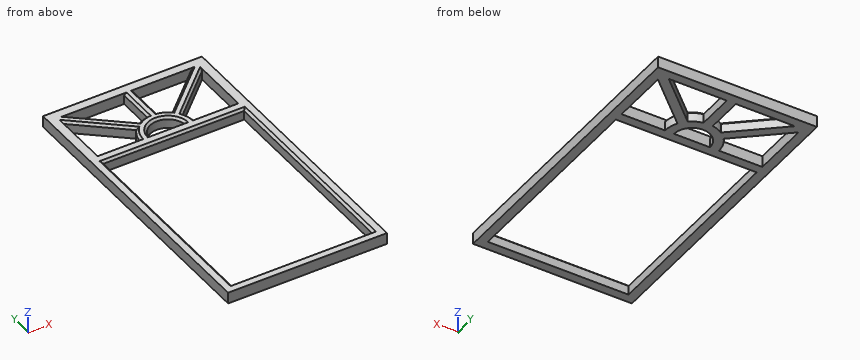
from build123d import *

# Parameters (mm, degrees)
F0_W     = 700
F0_H     = 1300
F0_W_2   = 620
F0_H_2   = 900
F1_DEPTH = 50
F2_SIZE  = 10


# Not quite as in the source:
# - a feature names something its author has since deleted; it is built from what else it names


with BuildPart() as f1:
    # F0 (on Top) → F1 (new body)
    with BuildSketch(Plane.XY):
        with Locations((-12.4809433535, 115.0203361814)):
            Rectangle(F0_W, F0_H)
        with Locations((-12.4809433535, -44.9796638186)):
            Rectangle(F0_W_2, F0_H_2, mode=Mode.SUBTRACT)
        Polygon((-131.3545905658, 445.0203361814), (-322.4809433535, 445.0203361814), (-322.4809433535, 700.0203361814), (-322.4809433535, 725.0203361814), (-290.108913989, 725.0203361814), (-30.108913989, 725.0203361814), (9.891086011, 725.0203361814), (265.6861508147, 725.0203361814), (297.5190566465, 725.0203361814), (297.5190566465, 700.0203361814), (297.5190566465, 445.0203361814), (106.3927038589, 445.0203361814), (66.3927038589, 445.0203361814), (-91.3545905658, 445.0203361814), align=None, mode=Mode.SUBTRACT)
        with BuildLine():
            Line((-322.4809433535, 725.0203361814), (-322.4809433535, 700.0203361814))
            Line((-322.4809433535, 700.0203361814), (-106.829258799, 517.3345075045))
            ThreePointArc((-106.829258799, 517.3345075045), (-93.2073200284, 532.2796973439), (-77.2493518889, 544.6998087791))
            Line((-77.2493518889, 544.6998087791), (-290.108913989, 725.0203361814))
            Line((-290.108913989, 725.0203361814), (-322.4809433535, 725.0203361814))
        make_face()
        with BuildLine():
            ThreePointArc((-106.829258799, 517.3345075045), (-125.0564121886, 483.2002761775), (-131.3545905658, 445.0203361814))
            Line((-131.3545905658, 445.0203361814), (-91.3545905658, 445.0203361814))
            ThreePointArc((-91.3545905658, 445.0203361814), (-12.4809433535, 523.8939833937), (66.3927038589, 445.0203361814))
            Line((66.3927038589, 445.0203361814), (106.3927038589, 445.0203361814))
            ThreePointArc((106.3927038589, 445.0203361814), (102.1362449296, 476.5456300205), (89.6716866284, 505.8132978575))
            ThreePointArc((89.6716866284, 505.8132978575), (77.9737439548, 522.1494068715), (63.691579675, 536.2819970091))
            ThreePointArc((63.691579675, 536.2819970091), (38.4127121689, 552.4483578012), (9.891086011, 561.7697957248))
            ThreePointArc((9.891086011, 561.7697957248), (-10.0745975152, 563.8696252044), (-30.108913989, 562.5796771664))
            ThreePointArc((-30.108913989, 562.5796771664), (-54.6379504639, 556.16767422), (-77.2493518889, 544.6998087791))
            ThreePointArc((-77.2493518889, 544.6998087791), (-93.2073200284, 532.2796973439), (-106.829258799, 517.3345075045))
        make_face()
        with BuildLine():
            Line((-30.108913989, 725.0203361814), (-30.108913989, 562.5796771664))
            ThreePointArc((-30.108913989, 562.5796771664), (-10.0745975152, 563.8696252044), (9.891086011, 561.7697957248))
            Line((9.891086011, 561.7697957248), (9.891086011, 725.0203361814))
            Line((9.891086011, 725.0203361814), (-30.108913989, 725.0203361814))
        make_face()
        with BuildLine():
            ThreePointArc((63.691579675, 536.2819970091), (77.9737439548, 522.1494068715), (89.6716866284, 505.8132978575))
            Line((89.6716866284, 505.8132978575), (297.5190566465, 700.0203361814))
            Line((297.5190566465, 700.0203361814), (297.5190566465, 725.0203361814))
            Line((297.5190566465, 725.0203361814), (265.6861508147, 725.0203361814))
            Line((265.6861508147, 725.0203361814), (63.691579675, 536.2819970091))
        make_face()
    extrude(amount=F1_DEPTH)

    # F2
    f2_edges = [f1.edges().sort_by_distance(p)[0] for p in [
        (-12.480943, 405.020336, 50),
        (297.519057, -44.979664, 50),
        (-12.480943, -494.979664, 50),
        (-322.480943, -44.979664, 50),
        (-12.480943, 523.893983, 50),
        (-54.63795, 556.167674, 50),
        (102.136245, 476.54563, 50),
        (-214.655101, 608.677422, 50),
        (-183.679133, 634.860072, 50),
        (-30.108914, 643.800007, 50),
        (38.412712, 552.448358, 50),
        (-125.056412, 483.200276, 50),
        (193.595372, 602.916817, 50),
        (164.688865, 630.651167, 50),
        (9.891086, 643.395066, 50),
    ]]
    chamfer(f2_edges, length=F2_SIZE)


solid = f1.part
Can you work these out from the model? Positions are in its coordinate system, mm. Give positions to 0.01 mm unless a question says otherwise; leave off trailing zeros. Order: outer loops, then holes, each group sorted by start corner. A loop starts at its lowest first (then second) coordinate and runs counter-clockwise, first axis right, second up. Notation, with made-up numbers: M 1.25,13.5 L 8.25,13.5 A19 cw 8.25,22.5 Z; hole C 81.5,-2.75 d7. An arc over 180 degrees is marked long. Use one line per item in the form item = value.
Item 1: If I drill on line 1 along X through (y, z) = (-181, 13); line 2 along Y through (x, z) = (-157, 41); line 3 along X through (y, z) = (677, 5), over which ranges is the centre line in solid material (lowest first)? Write a range as [from, to].
Values follow:
line_1 = [-362.48, -322.48], [297.52, 337.52]
line_2 = [-534.98, -495.98], [406.02, 445.02], [561.15, 610.95], [725.02, 765.02]
line_3 = [-362.48, -322.48], [-295.31, -233.42], [-30.11, 9.89], [214.29, 272.88], [297.52, 337.52]
Item 2: If we section it at A-A, the plane y = -110: Write out the boundary of the cut face in (x, z).
Values follow:
outline = M -362.48,0 L -322.48,0 L -322.48,40 L -332.48,50 L -362.48,50 Z; M 297.52,0 L 337.52,0 L 337.52,50 L 307.52,50 L 297.52,40 Z
Item 3: If we section it at C-C, the plane z = 29: Write out the boundary of the cut face in (x, y).
Values follow:
outline = M -362.48,-534.98 L 337.52,-534.98 L 337.52,765.02 L -362.48,765.02 Z; hole M -322.48,-494.98 L 297.52,-494.98 L 297.52,405.02 L -322.48,405.02 Z; hole M -322.48,445.02 L -131.35,445.02 A118.87 cw -106.83,517.33 L -322.48,700.02 Z; hole M -290.11,725.02 L -77.25,544.7 A118.87 cw -30.11,562.58 L -30.11,725.02 Z; hole M -91.35,445.02 L 66.39,445.02 A78.87 ccw Z; hole M 9.89,561.77 A118.87 cw 63.69,536.28 L 265.69,725.02 L 9.89,725.02 Z; hole M 89.67,505.81 A118.87 cw 106.39,445.02 L 297.52,445.02 L 297.52,700.02 Z
Item 4: If we section it at D-D, the plane x = 46: Count the separate pieces of the cut face and the enclosed holes in it, and give its area (3 significant figures).
Values follow:
separate_pieces = 4
enclosed_holes = 0
area = 8,300 mm^2
Item 5: If we section it at B-B, the plane x = -203: Write out the boundary of the cut face in (y, z), and give its area (3 significant figures).
Values follow:
outline = M -534.98,0 L -494.98,0 L -494.98,40 L -504.98,50 L -534.98,50 Z; M 405.02,0 L 445.02,0 L 445.02,50 L 415.02,50 L 405.02,40 Z; M 598.8,0 L 651.23,0 L 651.23,40 L 638.12,50 L 611.91,50 L 598.8,40 Z; M 725.02,0 L 765.02,0 L 765.02,50 L 725.02,50 Z
area = 8,390 mm^2
